```python
from build123d import *

# Parameters (mm, degrees)
ESQUISSE1_R                                        = 6.328378155
BOSS_EXTRU_1_DEPTH                                 = 70
ENL_V_MAT_EXTRU_3_DEPTH                            = 45
CONG_3_R                                           = 4
ESQUISSE5_R                                        = 20
ENL_V_MAT_EXTRU_4_DEPTH                            = 2
ESQUISSE6_R                                        = 10
ENL_V_MAT_EXTRU_5_DEPTH                            = 65
TROU_POUR_TARAUDAGE_POUR_TROU_TARAUD_M5_D          = 4.2
TROU_POUR_TARAUDAGE_POUR_TROU_TARAUD_M5_DEPTH      = 8
TROU_POUR_TARAUDAGE_POUR_TROU_TARAUD_M5_TIP        = 1.2618073
ENL_V_MAT_EXTRU_6_DEPTH                            = 45
CONG_5_R                                           = 4
ENL_V_MAT_EXTRU_7_DEPTH                            = 71
ENL_V_MAT_EXTRU_10_DEPTH                           = 30
ENL_V_MAT_EXTRU_10_DEPTH_BACK                      = 41
CHAMBRAGE_POUR_VIS_T_TE_HEXAGONALE_M51_D           = 5.5
CHAMBRAGE_POUR_VIS_T_TE_HEXAGONALE_M51_DEPTH       = 90
CHAMBRAGE_POUR_VIS_T_TE_HEXAGONALE_M51_CBORE_D     = 10
CHAMBRAGE_POUR_VIS_T_TE_HEXAGONALE_M51_CBORE_DEPTH = 40
CHAMBRAGE_POUR_VIS_T_TE_HEXAGONALE_M51_TIP         = 1.652366702
TROU_POUR_TARAUDAGE_POUR_TROU_TARAUD_M1_D          = 10.2
TROU_POUR_TARAUDAGE_POUR_TROU_TARAUD_M1_DEPTH      = 30
TROU_POUR_TARAUDAGE_POUR_TROU_TARAUD_M1_TIP        = 3.064389157
ESQUISSE20_R                                       = 6.5
ENL_V_MAT_EXTRU_11_DEPTH                           = 10
ENL_V_START                                        = -30
ENL_V_MAT_EXTRU_13_DEPTH                           = 45
CONG_9_R                                           = 2
TROU_POUR_TARAUDAGE_POUR_TROU_TARAUD_M4_D          = 3.3
TROU_POUR_TARAUDAGE_POUR_TROU_TARAUD_M4_DEPTH      = 8
TROU_POUR_TARAUDAGE_POUR_TROU_TARAUD_M4_TIP        = 0.991420021
CHANFREIN1_SIZE                                    = 0.5
D_GAGEMENT_M31_D                                   = 3.4
D_GAGEMENT_M31_DEPTH                               = 8
D_GAGEMENT_M31_TIP                                 = 1.021463052
ENL_V_MAT_EXTRU_25_DEPTH                           = 7
CONG_10_R                                          = 4
TROU_POUR_TARAUDAGE_POUR_TROU_TARAUD_M3_D          = 2.5
TROU_POUR_TARAUDAGE_POUR_TROU_TARAUD_M3_DEPTH      = 6
TROU_POUR_TARAUDAGE_POUR_TROU_TARAUD_M3_TIP        = 0.751075774


with BuildPart() as part:
    # Esquisse1 → Boss.-Extru.1 (new body)
    with BuildSketch(Plane.XY):
        Polygon((100, -50), (100, 50), (30, 50), (-40, 50), (-40, -50), (30, -50), align=None)
        Circle(ESQUISSE1_R, mode=Mode.SUBTRACT)
    extrude(amount=BOSS_EXTRU_1_DEPTH)

    # Esquisse9 → Enl_vement de mati_re-R_volution1 (revolve, cut)
    with BuildSketch(Plane(origin=(0, 0, 0), x_dir=(1, 0, 0), z_dir=(0, 1, 0))):
        Polygon((0, 0), (0, -70), (21.5, -70), (21.5, -58), (14, -58), (14, -45.8), (12.5, -45.8), (12.5, -18), (21, -18), (21, -6), (38, -6), (38, 0), align=None)
    revolve(axis=Axis((0, 0, 0), (0, 0, 1)), mode=Mode.SUBTRACT)

    # Esquisse4 → Enl_v. mat.-Extru.3 (cut)
    with BuildSketch(Plane(origin=(100, 0, 0), x_dir=(0, 0, -1), z_dir=(1, 0, 0))):
        Polygon((-65, -10.5), (-8, -10.5), (-8, 46.5), (-65, 46.5), (-70, 46.5), (-70, -10.5), align=None)
    extrude(amount=-ENL_V_MAT_EXTRU_3_DEPTH, mode=Mode.SUBTRACT)

    # Cong_3
    cong_3_edges = [part.edges().sort_by_distance(p)[0] for p in [
        (77.5, 46.5, 8),
        (77.5, -10.5, 8),
    ]]
    fillet(cong_3_edges, radius=CONG_3_R)

    # Esquisse5 → Enl_v. mat.-Extru.4 (cut)
    with BuildSketch(Plane(origin=(55, 0, 0), x_dir=(0, 0, -1), z_dir=(1, 0, 0))):
        with Locations((-36.8, 18)):
            Circle(ESQUISSE5_R)
    extrude(amount=-ENL_V_MAT_EXTRU_4_DEPTH, mode=Mode.SUBTRACT)

    # Esquisse6 → Enl_v. mat.-Extru.5 (cut)
    with BuildSketch(Plane(origin=(53, 0, 0), x_dir=(0, 0, -1), z_dir=(1, 0, 0))):
        with Locations((-36.8, 18)):
            Circle(ESQUISSE6_R)
    extrude(amount=-ENL_V_MAT_EXTRU_5_DEPTH, mode=Mode.SUBTRACT)

    # Trou pour taraudage pour trou taraud_ M5
    with Locations(Plane(origin=(55, 0, 0), x_dir=(0, 0, -1), z_dir=(1, 0, 0))):
        with Locations((-36.8, 18), (-13.23, 41.57), (-60.37, -5.57), (-60.37, 41.57), (-13.23, -5.57)):
            Hole(TROU_POUR_TARAUDAGE_POUR_TROU_TARAUD_M5_D / 2, depth=TROU_POUR_TARAUDAGE_POUR_TROU_TARAUD_M5_DEPTH)
            with Locations((0, 0, -(TROU_POUR_TARAUDAGE_POUR_TROU_TARAUD_M5_DEPTH + TROU_POUR_TARAUDAGE_POUR_TROU_TARAUD_M5_TIP / 2))):  # 118° drill point
                Cone(0, TROU_POUR_TARAUDAGE_POUR_TROU_TARAUD_M5_D / 2, TROU_POUR_TARAUDAGE_POUR_TROU_TARAUD_M5_TIP, mode=Mode.SUBTRACT)

    # Esquisse10 → Enl_v. mat.-Extru.6 (cut)
    with BuildSketch(Plane(origin=(100, 0, 0), x_dir=(0, 0, -1), z_dir=(1, 0, 0))):
        Polygon((-13, -38), (-70, -38), (-70, -2.141745164), (-8, -2.141745164), (-8, -33), align=None)
    extrude(amount=-ENL_V_MAT_EXTRU_6_DEPTH, mode=Mode.SUBTRACT)

    # Cong_5
    cong_5_edges = [part.edges().sort_by_distance(p)[0] for p in [
        (77.5, -33, 8),
        (77.5, -38, 13),
    ]]
    fillet(cong_5_edges, radius=CONG_5_R)

    # Esquisse11 → Enl_v. mat.-Extru.7 (cut, through all)
    with BuildSketch(Plane(origin=(0, 0, 0), x_dir=(-1, 0, 0), z_dir=(0, 0, -1))):
        with BuildLine():
            Line((40, -50), (40, -1.07e-07))
            ThreePointArc((40, -1.07e-07), (31.887007625, -24.149922251), (10.839062865, -38.503437719))
            Line((10.839062865, -38.503437719), (-30, -50))
            Line((-30, -50), (40, -50))
        make_face()
        with BuildLine():
            Line((40, 50), (-30, 50))
            Line((-30, 50), (10.839062865, 38.503437719))
            ThreePointArc((10.839062865, 38.503437719), (31.887007689, 24.149922166), (40, -1.07e-07))
            Line((40, -1.07e-07), (40, 50))
        make_face()
    extrude(amount=-ENL_V_MAT_EXTRU_7_DEPTH, mode=Mode.SUBTRACT)

    # Esquisse14 → Enl_v. mat.-Extru.10 (cut, two sides)
    with BuildSketch(Plane(origin=(0, 0, 0), x_dir=(0, 0, -1), z_dir=(1, 0, 0))) as enl_v_mat_extru_10_sk:
        with BuildLine():
            Line((-17.774653975, 50), (-58.226182617, 31.13714241))
            ThreePointArc((-58.226182617, 31.13714241), (-62.433914458, 27.447060623), (-64, 22.074064539))
            Line((-64, 22.074064539), (-64, -22.074064539))
            ThreePointArc((-64, -22.074064539), (-62.433914458, -27.447060623), (-58.226182617, -31.13714241))
            Line((-58.226182617, -31.13714241), (-17.774653975, -50))
            Line((-17.774653975, -50), (-70, -50))
            Line((-70, -50), (-70, 50))
            Line((-70, 50), (-17.774653975, 50))
        make_face()
    extrude(amount=ENL_V_MAT_EXTRU_10_DEPTH, mode=Mode.SUBTRACT)
    extrude(enl_v_mat_extru_10_sk.sketch, amount=-ENL_V_MAT_EXTRU_10_DEPTH_BACK, mode=Mode.SUBTRACT)

    # Chambrage pour vis _ t_te hexagonale M51
    with Locations(Plane(origin=(0, 0, 0), x_dir=(-1, 0, 0), z_dir=(0, 0, -1))):
        with Locations((-85, -44), (-36, -44), (-36, 44)):
            CounterBoreHole(CHAMBRAGE_POUR_VIS_T_TE_HEXAGONALE_M51_D / 2, CHAMBRAGE_POUR_VIS_T_TE_HEXAGONALE_M51_CBORE_D / 2, CHAMBRAGE_POUR_VIS_T_TE_HEXAGONALE_M51_CBORE_DEPTH, depth=CHAMBRAGE_POUR_VIS_T_TE_HEXAGONALE_M51_DEPTH)
            with Locations((0, 0, -(CHAMBRAGE_POUR_VIS_T_TE_HEXAGONALE_M51_DEPTH + CHAMBRAGE_POUR_VIS_T_TE_HEXAGONALE_M51_TIP / 2))):  # 118° drill point
                Cone(0, CHAMBRAGE_POUR_VIS_T_TE_HEXAGONALE_M51_D / 2, CHAMBRAGE_POUR_VIS_T_TE_HEXAGONALE_M51_TIP, mode=Mode.SUBTRACT)

    # Trou pour taraudage pour trou taraud_ M1
    with Locations(Plane(origin=(0, 0, 0), x_dir=(-1, 0, 0), z_dir=(0, 0, -1))):
        with Locations((-43.301270189, -25)):
            Hole(TROU_POUR_TARAUDAGE_POUR_TROU_TARAUD_M1_D / 2, depth=TROU_POUR_TARAUDAGE_POUR_TROU_TARAUD_M1_DEPTH)
            with Locations((0, 0, -(TROU_POUR_TARAUDAGE_POUR_TROU_TARAUD_M1_DEPTH + TROU_POUR_TARAUDAGE_POUR_TROU_TARAUD_M1_TIP / 2))):  # 118° drill point
                Cone(0, TROU_POUR_TARAUDAGE_POUR_TROU_TARAUD_M1_D / 2, TROU_POUR_TARAUDAGE_POUR_TROU_TARAUD_M1_TIP, mode=Mode.SUBTRACT)

    # Esquisse20 → Enl_v. mat.-Extru.11 (cut)
    with BuildSketch(Plane(origin=(0, 0, 0), x_dir=(-1, 0, 0), z_dir=(0, 0, -1))):
        with Locations((-43.301270189, -25)):
            Circle(ESQUISSE20_R)
    extrude(amount=-ENL_V_MAT_EXTRU_11_DEPTH, mode=Mode.SUBTRACT)

    # Esquisse24 → Enl_v. mat.-Extru.13 (cut)
    with BuildSketch(Plane(origin=(0, 0, 0), x_dir=(-1, 0, 0), z_dir=(0, 0, -1)).offset(ENL_V_START)):
        with BuildLine():
            Line((-43.301270189, -10), (-55, -10))
            Line((-55, -10), (-55, -38))
            Line((-55, -38), (-43.301270189, -38))
            ThreePointArc((-43.301270189, -38), (-36.230202377, -35.071067812), (-33.301270189, -28))
            Line((-33.301270189, -28), (-33.301270189, -20))
            ThreePointArc((-33.301270189, -20), (-36.230202377, -12.928932188), (-43.301270189, -10))
        make_face()
    extrude(amount=-ENL_V_MAT_EXTRU_13_DEPTH, mode=Mode.SUBTRACT)

    # Cong_9
    cong_9_edges = [part.edges().sort_by_distance(p)[0] for p in [
        (55, -10, 50),
    ]]
    fillet(cong_9_edges, radius=CONG_9_R)

    # Trou pour taraudage pour trou taraud_ M4
    with Locations(Plane(origin=(100, 0, 0), x_dir=(0, 0, -1), z_dir=(1, 0, 0))):
        with Locations((-5, -44), (-5, 44)):
            Hole(TROU_POUR_TARAUDAGE_POUR_TROU_TARAUD_M4_D / 2, depth=TROU_POUR_TARAUDAGE_POUR_TROU_TARAUD_M4_DEPTH)
            with Locations((0, 0, -(TROU_POUR_TARAUDAGE_POUR_TROU_TARAUD_M4_DEPTH + TROU_POUR_TARAUDAGE_POUR_TROU_TARAUD_M4_TIP / 2))):  # 118° drill point
                Cone(0, TROU_POUR_TARAUDAGE_POUR_TROU_TARAUD_M4_D / 2, TROU_POUR_TARAUDAGE_POUR_TROU_TARAUD_M4_TIP, mode=Mode.SUBTRACT)

    # Chanfrein1
    chanfrein1_edges = [part.edges().sort_by_distance(p)[0] for p in [
        (9.580468567, 44.25171886, 0),
        (-40, 0, 0),
        (9.580468567, -44.25171886, 0),
        (65, -50, 0),
        (65, 50, 0),
        (-12.5, 0, 18),
        (-21, 0, 6),
        (-38, 0, 0),
        (30, -50, 43.887326987),
        (30, 50, 43.887326987),
    ]]
    chamfer(chanfrein1_edges, length=CHANFREIN1_SIZE)

    # D_gagement M31
    with Locations(Plane.XY.offset(58)):
        with Locations((-17, 0), (8.5, 14.722431864), (8.5, -14.722431864), (0, 0)):
            Hole(D_GAGEMENT_M31_D / 2, depth=D_GAGEMENT_M31_DEPTH)
            with Locations((0, 0, -(D_GAGEMENT_M31_DEPTH + D_GAGEMENT_M31_TIP / 2))):  # 118° drill point
                Cone(0, D_GAGEMENT_M31_D / 2, D_GAGEMENT_M31_TIP, mode=Mode.SUBTRACT)

    # Esquisse32 → Enl_v. mat.-Extru.25 (cut)
    with BuildSketch(Plane(origin=(100, 0, 0), x_dir=(0, 0, -1), z_dir=(1, 0, 0))):
        with BuildLine():
            ThreePointArc((-8, -31.343145751), (-8.30448187, -32.87387948), (-9.171572875, -34.171572875))
            Line((-9.171572875, -34.171572875), (-2, -27))
            Line((-2, -27), (-2, -13.8))
            Line((-2, -13.8), (-8, -13.8))
            Line((-8, -13.8), (-8, -31.343145751))
        make_face()
        with BuildLine():
            Line((-70, -38), (-70, -47))
            Line((-70, -47), (-22, -47))
            Line((-22, -47), (-11.828427125, -36.828427125))
            ThreePointArc((-11.828427125, -36.828427125), (-13.12612052, -37.69551813), (-14.656854249, -38))
            Line((-14.656854249, -38), (-70, -38))
        make_face()
    extrude(amount=-ENL_V_MAT_EXTRU_25_DEPTH, mode=Mode.SUBTRACT)

    # Cong_10
    cong_10_edges = [part.edges().sort_by_distance(p)[0] for p in [
        (96.5, -27, 2),
        (96.5, -13.8, 2),
        (96.5, -47, 22),
    ]]
    fillet(cong_10_edges, radius=CONG_10_R)

    # Trou pour taraudage pour trou taraud_ M3
    with Locations(Plane(origin=(93, 0, 0), x_dir=(0, 0, -1), z_dir=(1, 0, 0))):
        with Locations((-5.5, -20), (-51.8, -40.5)):
            Hole(TROU_POUR_TARAUDAGE_POUR_TROU_TARAUD_M3_D / 2, depth=TROU_POUR_TARAUDAGE_POUR_TROU_TARAUD_M3_DEPTH)
            with Locations((0, 0, -(TROU_POUR_TARAUDAGE_POUR_TROU_TARAUD_M3_DEPTH + TROU_POUR_TARAUDAGE_POUR_TROU_TARAUD_M3_TIP / 2))):  # 118° drill point
                Cone(0, TROU_POUR_TARAUDAGE_POUR_TROU_TARAUD_M3_D / 2, TROU_POUR_TARAUDAGE_POUR_TROU_TARAUD_M3_TIP, mode=Mode.SUBTRACT)


solid = part.part
```
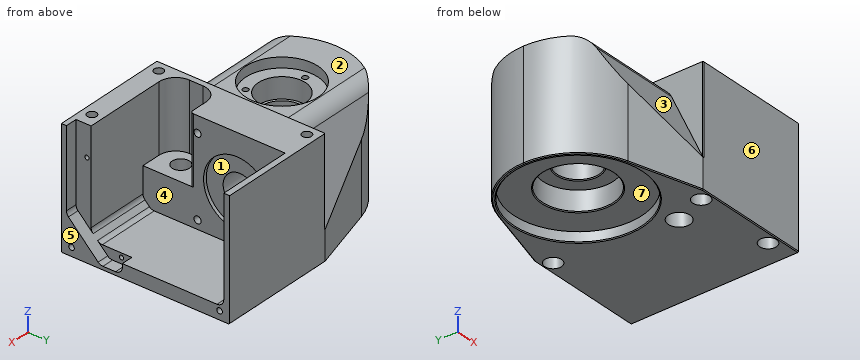
For this review, take the finished solid that the model builds, in its own axes (mm). Face numbers are marked on the shaded views. A direction names the side the tool comes from. Round coordinates to 2 decimals unless told otherwise and drop trailing zeros. Write each loop counter-clockwise with the first axis right and the second up, starting at its lowest first coordinate (ties: lowest second). Pieces come first, ordered by that corner, then holes. Notation, with made-up numbers: (11.25, -11) -> (28.25, -11) arc R16 cw to (28.25, 6) -> close; hole circle Ø9 at (-2.5, 53.25). An arc over 180 degrees is marked (long way). One line per question, with ' | ' between items. Start each with the question number.
1) Add section B-B (z = 36.5). Count the separate pieces of the cut face and the enclosed holes in it, and give its area (3 significant figures).
2) Add section A-A (x = 72). Write out the cut boundary in (y, z), and give its area (3 significant figures).
3) Wall thickness on line 1 along Y through (x, z) = (89.95, 51.8); line 2 along Y through (x, z) = (77.5, 30.5); line 3 along Z through (x, y) = (49, 41.57): over which ranges is each line inside the solid? List them lowest first.
4) For pin 1 Ø13 at (x, y) = (-1, -6.5) entering from +Z; pin 2 Ø6 at (y, z) = (-26, 56) entering from -X; pin 3 Ø1.5 at (y, z) = (-10, 55.5) entering from +X, all flat-tipped, find the tip position at first contact; note any pin that passes through.
5) Mouldability with a two-part tool opening along Y and no side actions: class the marked faces 4, 5, 6 and 7 as +Y half, -Y half, draft (parallel to the pull), parting line (faces both ways), or undercut.
6) Machinability: for the marked faces 1, 2 and 3, which of the approach directions +Z, -Z, +X, -X, +Y, -Y give a long, thin tool a straight path to every point of the face, cutting with its end or side? Answer none if there is none.
Reported:
1) separate pieces: 1 | enclosed holes: 3 | area: 5,520 mm²
2) outline: (-50, 0.5) -> (-49.5, 0) -> (49.5, 0) -> (50, 0.5) -> (50, 70) -> (46.5, 70) -> (46.5, 12) arc R4 cw to (42.5, 8) -> (-31.34, 8) arc R4 cw to (-34.17, 9.17) -> (-36.83, 11.83) arc R4 cw to (-38, 14.66) -> (-38, 70) -> (-50, 70) -> close | area: 1,780 mm²
3) line 1: y = -50 to -41.75, -39.25 to -38, 46.5 to 50 | line 2: y = -50 to -38, 46.5 to 50 | line 3: z = 0 to 11.13, 15.33 to 58.27, 62.47 to 70
4) pin 1: stops at z = 45.8 | pin 2: stops at x = -32.73 | pin 3: stops at x = 54.56
5) face 4: undercut | face 5: draft | face 6: -Y half | face 7: undercut
6) face 1: +X | face 2: +Z, -X, +Y, -Y | face 3: +Z, -X, -Y
